Read the model definition and answer for the solid it produces. Units are mm, in the model's axes. A direction names the side the tool comes from. Round coordinates to 2 decimals unless told otherwise and drop trailing zeros. Loops run counter-clockwise (first coordinate to the right, second up) from the corner with the lowest first, then second, coordinate; pieces in that order, holes last. Notation, with made-up numbers: (70, 0) - (113, 0) arc R36 ccw to (113, 34) - close; hole circle Ø11 at (-0.75, -36). An arc over 180 degrees is marked (long way). Use CSV: the item, a comma, the result in double quotes. Start each with the question number.
1. Find section B-B (x = 0). Give the vertices of the cut face in (y, z).
2. Determine the mould class of faces 3 (the flat face through (1, 0, -1)), 4 (the flat face through (-23, -22, -0.5)), 5 (the cylindrical face through (-9.051, -19.151, 40.757)) for opening direction X: +X half, -X half, draft (parallel to the pull), parting line (faces both ways), or undercut.
3. Consider line 1 along Y through (x, z) = (13.5, -36.5); line 2 along Z through (x, y) = (27, -38); line 3 along X through (y, z) = (-26.1, 15.5). Determine where each line is inside the solid, lowest interval first.
4. A tool of negligible diameter and unlimited length cuts with its end or side. For faces 1 (the flat face through (-25, -31, -11.95)), 2 (the flat face through (-28, -34.5, -15)), from which of +Z, -Z, +X, -X, +Y, -Y can it reach the whole face along a straight path? Write none if from no direction.
5. Find section A-A (y = -24.5). State how many separate pieces and enclosed holes the cut face has, and give its area (3 significant figures).
6. Given pin 1 Ø6 at (x, z) = (8.5, 11) entering from -Y; pin 2 Ø5 at (x, y) = (-10.5, -27) entering from +Z; pin 3 Ø5 at (x, y) = (28, -13.5) entering from -Z, each flat-ended and moving along its own axis, determine where each tip first touches the part or whether it passes through.
from build123d import *

# Parameters (mm, degrees)
CUT_EXTRUDE1_DEPTH       = 37
SKETCH3_R                = 4
CUT_EXTRUDE2_DEPTH       = 37
SKETCH4_W                = 72
SKETCH4_H                = 1
CUT_EXTRUDE3_DEPTH       = 37
M4_CLEARANCE_HOLE1_D     = 4.5
M4_CLEARANCE_HOLE1_DEPTH = 18
M4_CLEARANCE_HOLE1_TIP   = 1.351936393
CUT_EXTRUDE4_START       = -6
CUT_EXTRUDE4_DEPTH       = 6
SKETCH8_R                = 2.25
BOSS_EXTRUDE1_DEPTH      = 0.5


with BuildPart() as part:
    # Sketch1 → Revolve1 (revolve)
    with BuildSketch(Plane.XY, mode=Mode.PRIVATE) as revolve1_sk:
        Polygon((0, 0), (-41.75, 0), (-41.75, -5), (-37.5, -5), (-37.5, -13), (-41.75, -17.25), (-41.75, -21), (-37.5, -21), (-37.5, -29), (-41.75, -33.25), (-41.75, -40), (0, -40), align=None)
    revolve(revolve1_sk.sketch.rotate(Axis((0, -40, 0), (0, 1, 0)), 180), axis=Axis((0, -40, 0), (0, 1, 0)))

    # Sketch2 → Cut-Extrude1 (cut)
    with BuildSketch(Plane(origin=(0, -40, 0), x_dir=(1, 0, 0), z_dir=(0, 1, 0))):
        Polygon((-21.5, 21.5), (-5, 21.5), (-5, 26.5), (5, 26.5), (5, 21.5), (21.5, 21.5), (21.5, -21.5), (-21.5, -21.5), align=None)
    extrude(amount=CUT_EXTRUDE1_DEPTH, mode=Mode.SUBTRACT)

    # Sketch3 → Cut-Extrude2 (cut)
    with BuildSketch(Plane.XZ.offset(40)):
        with Locations((-27.5, 0)):
            Circle(SKETCH3_R)
        with Locations((27.5, 0)):
            Circle(SKETCH3_R)
    extrude(amount=-CUT_EXTRUDE2_DEPTH, mode=Mode.SUBTRACT)

    # Sketch4 → Cut-Extrude3 (cut)
    with BuildSketch(Plane.XZ.offset(40)):
        Rectangle(SKETCH4_W, SKETCH4_H)
    extrude(amount=-CUT_EXTRUDE3_DEPTH, mode=Mode.SUBTRACT)

    # M4 Clearance Hole1
    with Locations(Plane(origin=(0, -40, 0), x_dir=(-1, 0, 0), z_dir=(0, -1, 0))):
        with Locations((27.5, -15.5), (-27.5, -15.5), (-27.5, 15.5), (27.5, 15.5)):
            Hole(M4_CLEARANCE_HOLE1_D / 2, depth=M4_CLEARANCE_HOLE1_DEPTH)
            with Locations((0, 0, -(M4_CLEARANCE_HOLE1_DEPTH + M4_CLEARANCE_HOLE1_TIP / 2))):  # 118° drill point
                Cone(0, M4_CLEARANCE_HOLE1_D / 2, M4_CLEARANCE_HOLE1_TIP, mode=Mode.SUBTRACT)

    # Sketch7 → Cut-Extrude4 (cut)
    with BuildSketch(Plane.XZ.offset(40).offset(CUT_EXTRUDE4_START)):
        Polygon((-25.450406544, 19.05), (25.450406544, 19.05), (29.549593456, 19.05), (31.599186911, 15.5), (29.549593456, 11.95), (25.450406544, 11.95), (-25.450406544, 11.95), (-29.549593456, 11.95), (-31.599186911, 15.5), (-29.549593456, 19.05), align=None)
        Polygon((25.450406544, -11.95), (-25.450406544, -11.95), (-29.549593456, -11.95), (-31.599186911, -15.5), (-29.549593456, -19.05), (-25.450406544, -19.05), (25.450406544, -19.05), (29.549593456, -19.05), (31.599186911, -15.5), (29.549593456, -11.95), align=None)
    extrude(amount=-CUT_EXTRUDE4_DEPTH, mode=Mode.SUBTRACT)

    # Sketch8 → Boss-Extrude1 (add)
    with BuildSketch(Plane(origin=(0, -34, 0), x_dir=(1, 0, 0), z_dir=(0, 1, 0))):
        with Locations(Location((-27.5, -15.5, 0), (0, 0, 90))):
            Circle(SKETCH8_R)
        with Locations(Location((-27.5, 15.5, 0), (0, 0, 90))):
            Circle(SKETCH8_R)
        with Locations(Location((27.5, 15.5, 0), (0, 0, 90))):
            Circle(SKETCH8_R)
        with Locations(Location((27.5, -15.5, 0), (0, 0, 90))):
            Circle(SKETCH8_R)
    extrude(amount=-BOSS_EXTRUDE1_DEPTH)


solid = part.part
Filled sheet:
1,outline,"(-40, -41.75) - (-33.25, -41.75) - (-29, -37.5) - (-21, -37.5) - (-21, -41.75) - (-17.25, -41.75) - (-13, -37.5) - (-5, -37.5) - (-5, -41.75) - (0, -41.75) - (0, 41.75) - (-5, 41.75) - (-5, 37.5) - (-13, 37.5) - (-17.25, 41.75) - (-21, 41.75) - (-21, 37.5) - (-29, 37.5) - (-33.25, 41.75) - (-40, 41.75) - (-40, 21.5) - (-3, 21.5) - (-3, -26.5) - (-40, -26.5) - close"
2,face 3,"draft"
2,face 4,"undercut"
2,face 5,"parting line"
3,line 1,"y = -40 to -30.42, -21 to -14.42, -5 to 0"
3,line 2,"z = -31.84 to -17.69, -13.31 to -3.97, 3.97 to 13.31, 17.69 to 31.84"
3,line 3,"x = -34.15 to -29.75, -25.25 to -21.5, 21.5 to 25.25, 29.75 to 34.15"
4,face 1,"none"
4,face 2,"-Y"
5,separate pieces,"1"
5,enclosed holes,"5"
5,area,"2,340 mm²"
6,pin 1,"stops at y = -3"
6,pin 2,"stops at z = 36.64"
6,pin 3,"stops at z = -29.97"
